Design review of the part built by this model. Coordinates are the model's own, in mm. A direction names the side the tool comes from. Coordinates: 2 decimals unless noted, no trailing zeros. Write each loop counter-clockwise with the first axis right and the second up, starting at its lowest first coordinate (ties: lowest second). Pieces come first, ordered by that corner, then holes.
Q1. For probe 1 along X at (y, z) = (-0.65, 20.5); probe 2 along Y at (x, z) = (5, 10) (3 decimals); probe 3 along Z at (x, y) = (4.5, -2), list the stretches that pass through material, from the lowest coordinate up.
Q2. Mouldability with a two-part tool opening along Z and no side actions: class faces 1 (the flat face through (43.307, -1, 11)), 2 (the cylindrical face through (1.81, -2.58, 1.91)), 3 (the flat face through (22, -1, 26.314)) as pulls with the +Z half, pulls with the -Z half, needs draft (parallel to the pull), parting line crosses it, or undercut.
Q3. Insertion check: pin 1 (3 mm diameter, centred on x = 41.25, z = 33.17, fed in from -Y); pin 2 (0.6 mm diameter, centred on x = 40, y = -0.5, fed in from -Z); pin 3 (0.6 mm diameter, centred on y = -0.5, z = 19.5, fed in from +X). Each pin has a flat end and moves straight along its axis. Give the tip position at first contact, or say it passes through.
Q4. Take a section at D-D (y = -4.5). State how many separate pieces and enclosed holes the cut face has, and give its area (3 significant figures).
Q5. Machinability: for faces 4 (the flat face through (31, -2, 42.24)), 5 (the flat face through (40, -1, 16.51)), 6 (the flat face through (22, -1, 16.993)), which of the approach directions +Z, -Z, +X, -X, +Y, -Y give a long, thin tool a straight path to every point of the face, cutting with its end or side? Answer none if there is none.
Q6. Take a section at C-C (x = 34). Give the boundary of the cut face in (y, z) (3 decimals).
Q7. Take a section at A-A (x = 21). Give the boundary of the cut face in (y, z) (3 decimals).
Q8. Take a section at B-B (z = 22). Give the boundary of the cut face in (x, y) (1 decimal), and give its area (3 significant figures).
```python
from build123d import *

# Parameters (mm, degrees)
F0_W         = 43.307
F0_H         = 43.307
F1_DEPTH     = 1.27
F3_DEPTH     = 3.175
F5_DEPTH     = 1.905
F6_R         = 0.889
F7_DEPTH     = 5.081
F8_W         = 9.3218
F8_H         = 9.3218
F8_W_2       = 7.0612
F8_H_2       = 10.3124
F10_DEPTH    = 1.27
F11_D        = 3.175
F14_D        = 2.54
F15_R        = 6.35
F16_T4_DEPTH = 12.7851645967
F16_T9_DEPTH = 12.8907938144
F17_R        = 0.7874
F18_D        = 3.175
F18_DEPTH    = 3.175
F18_TIP      = 0.9538662327


# Not quite as in the source:
# - a fillet or chamfer that OpenCascade refuses, or shapes differently, is made with other operations: its cross-section is extruded or revolved along the edge and cut away or added


with BuildPart() as f1:
    # F0 (on Front) → F1 (new body)
    with BuildSketch(Plane.XZ):
        with Locations((21.6535, 21.6535)):
            Rectangle(F0_W, F0_H)
    extrude(amount=F1_DEPTH)

    # F2 (on Front) → F3 (join)
    with BuildSketch(Plane.XZ):
        with BuildLine():
            Line((43.307, 43.307), (0, 43.307))
            Line((0, 43.307), (0, 0))
            Line((0, 0), (43.307, 0))
            Line((43.307, 0), (43.307, 1.0922))
            Line((43.307, 1.0922), (21.6408, 1.0922))
            ThreePointArc((21.6408, 1.0922), (1.0668, 21.6662), (21.6408, 42.2402))
            Line((21.6408, 42.2402), (43.307, 42.2402))
            Line((43.307, 42.2402), (43.307, 43.307))
        make_face()
    extrude(amount=F3_DEPTH)

    # F4 (on face) → F5 (join)
    with BuildSketch(Plane.XZ.offset(3.175)):
        with BuildLine():
            Line((43.307, 43.307), (0, 43.307))
            Line((0, 43.307), (0, 0))
            Line((0, 0), (43.307, 0))
            Line((43.307, 0), (43.307, 2.54))
            Line((43.307, 2.54), (21.6408, 2.54))
            ThreePointArc((21.6408, 2.54), (2.5146, 21.6662), (21.6408, 40.7924))
            Line((21.6408, 40.7924), (43.307, 40.7924))
            Line((43.307, 40.7924), (43.307, 43.307))
        make_face()
    extrude(amount=F5_DEPTH)

    # F6 (on face) → F7 (cut, through all)
    with BuildSketch(Plane(origin=(0, 0, 0), x_dir=(-1, 0, 0), z_dir=(0, 1, 0))):
        with Locations((-41.2496, 33.1724)):
            Circle(F6_R)
        with Locations((-2.667, 33.1724)):
            Circle(F6_R)
        with Locations((-41.2496, 10.16)):
            Circle(F6_R)
        with Locations((-2.667, 10.16)):
            Circle(F6_R)
    extrude(amount=-F7_DEPTH, mode=Mode.SUBTRACT)

    # F8 (on face) → F10 (cut, through all)
    with BuildSketch(Plane.XZ.offset(1.27)):
        with Locations((21.6535, 21.6535)):
            Rectangle(F8_W, F8_H)
        with Locations((39.7764, 21.6662)):
            Rectangle(F8_W_2, F8_H_2)
    extrude(amount=-F10_DEPTH, mode=Mode.SUBTRACT)

    # F11 (through all)
    with Locations(Plane(origin=(0, 0, 0), x_dir=(-1, 0, 0), z_dir=(0, 1, 0))):
        with Locations((-4.0894, 39.2176), (-4.0894, 4.0894)):
            Hole(F11_D / 2)

    # F14 (through all)
    with Locations(Plane(origin=(0, 0, 0), x_dir=(-1, 0, 0), z_dir=(0, 1, 0))):
        with Locations((-21.6535, 32.1564), (-21.6535, 11.176)):
            Hole(F14_D / 2)

    # F15
    f15_edges = [f1.edges().sort_by_distance(p)[0] for p in [
        (0, -2.54, 43.307),
        (43.307, -2.54, 43.307),
        (43.307, -2.54, 0),
        (0, -2.54, 0),
    ]]
    fillet(f15_edges, radius=F15_R)

    # F16: fillet of radius 0.8128 on 2 edges, made by hand


with BuildPart() as f16_tool2:
    # F16_s3 → F16_t4 (new body)
    with BuildSketch(Plane.XZ.offset(10.5200822984)):
        with BuildLine():
            ThreePointArc((40.005, 2.54), (40.7835212046, 1.9607563614), (40.452412844, 1.0486238532))
            ThreePointArc((40.452412844, 1.0486238532), (41.3090658387, 1.7259300464), (42.037, 2.54))
            Line((42.037, 2.54), (40.005, 2.54))
        make_face()
    extrude(amount=-F16_T4_DEPTH)

    split(bisect_by=Plane.XZ.offset(1.27), keep=Keep.TOP)


with BuildPart() as f1_1:
    add(f1.part)

    # F16_t1: cut F16_tool2
    add(f16_tool2.part, mode=Mode.SUBTRACT)


with BuildPart() as f16_tool7:
    # F16_s8 → F16_t9 (new body)
    with BuildSketch(Plane.XZ.offset(10.5728969072)):
        with BuildLine():
            ThreePointArc((39.9661228955, 40.7924), (40.7456166441, 41.374910322), (40.4078290086, 42.2875045872))
            ThreePointArc((40.4078290086, 42.2875045872), (41.2779959557, 41.6101165847), (42.0178504068, 40.7924))
            Line((42.0178504068, 40.7924), (39.9661228955, 40.7924))
        make_face()
    extrude(amount=-F16_T9_DEPTH)

    split(bisect_by=Plane.XZ.offset(1.27), keep=Keep.TOP)


with BuildPart() as f1_2:
    add(f1_1.part)

    # F16_t6: cut F16_tool7
    add(f16_tool7.part, mode=Mode.SUBTRACT)

    # F17
    f17_edges = [f1_2.edges().sort_by_distance(p)[0] for p in [
        (43.307, -0.635, 26.8224),
        (36.2458, -0.635, 26.8224),
        (16.9926, -0.635, 26.3144),
        (16.9926, -0.635, 16.9926),
        (26.3144, -0.635, 16.9926),
        (43.307, -0.635, 16.51),
        (36.2458, -0.635, 16.51),
        (26.3144, -0.635, 26.3144),
    ]]
    fillet(f17_edges, radius=F17_R)

    # F18
    with Locations(Plane(origin=(0, 0, 0), x_dir=(-1, 0, 0), z_dir=(0, 1, 0))):
        with Locations((-39.2176, 4.0894), (-39.2176, 39.2176)):
            Hole(F18_D / 2, depth=F18_DEPTH)
            with Locations((0, 0, -(F18_DEPTH + F18_TIP / 2))):  # 118° drill point
                Cone(0, F18_D / 2, F18_TIP, mode=Mode.SUBTRACT)


solid = f1_2.part
```
Response:
1. probe 1: x = 0 to 16.99, 26.31 to 36.25
1. probe 2: y = -5.08 to -3.175, -1.27 to 0
1. probe 3: z = 0.28 to 2.56, 5.62 to 10.29, 33.05 to 37.68, 40.75 to 43.03
2. face 1: needs draft
2. face 2: pulls with the -Z half
2. face 3: undercut
3. pin 1: stops at y = -1.27
3. pin 2: stops at z = 0.62
3. pin 3: stops at x = 36.25
4. separate pieces: 1
4. enclosed holes: 4
4. area: 418 mm2
5. face 4: +X
5. face 5: +X, +Y, -Y
5. face 6: +Y, -Y
6. outline: (-5.08, 0) - (0, 0) - (0, 43.307) - (-5.08, 43.307) - (-5.08, 40.792) - (-3.175, 40.792) - (-3.175, 42.24) - (-1.27, 42.24) - (-1.27, 1.092) - (-3.175, 1.092) - (-3.175, 2.54) - (-5.08, 2.54) - close
7. outline: (-5.08, 0) - (0, 0) - (0, 10.087) - (-1.27, 10.087) - (-1.27, 1.102) - (-3.175, 1.102) - (-3.175, 2.551) - (-5.08, 2.551) - close; (-5.08, 40.782) - (-3.175, 40.782) - (-3.175, 42.23) - (-1.27, 42.23) - (-1.27, 33.245) - (0, 33.245) - (0, 43.307) - (-5.08, 43.307) - close; (-1.27, 12.265) - (0, 12.265) - (0, 16.993) - (-1.27, 16.993) - close; (-1.27, 26.314) - (0, 26.314) - (0, 31.067) - (-1.27, 31.067) - close
8. outline: (0, -5.1) - (2.5, -5.1) - (2.5, -3.2) - (1.1, -3.2) - (1.1, -1.3) - (17, -1.3) - (17, 0) - (0, 0) - close; (26.3, -1.3) - (36.2, -1.3) - (36.2, 0) - (26.3, 0) - close
8. area: 41.0 mm2
